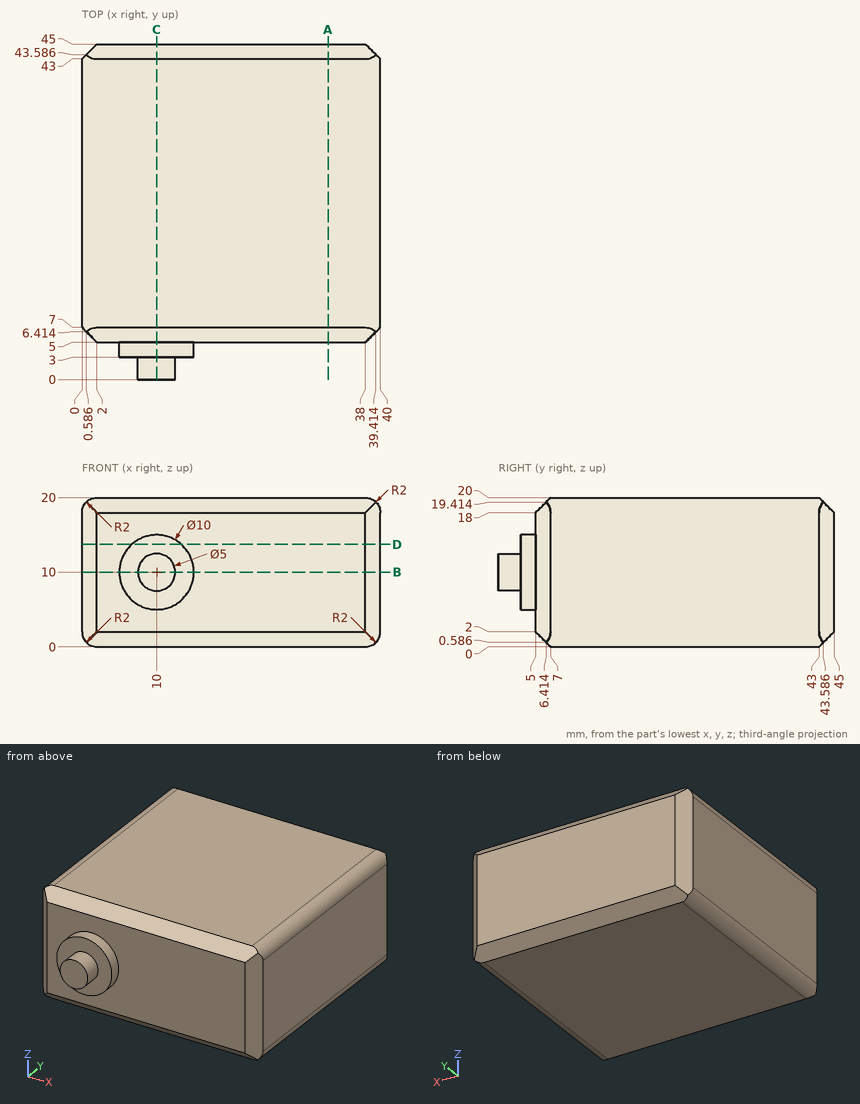
Input: dimensioned drawing with shaded views. Units: mm. Origin: part minimum x, y, z. Give positions to 0.01 mm unless a question says otherwise; leave off trailing zeros. Order: outer loops, then holes, each group sorted by start corner. A loop starts at its lowest first (then second) coordinate and runs counter-clockwise, first axis right, second up.
(1) Material intervals for line 1 along Y through (x, z) = (29.5, 17.75); line 2 along Y through (x, z) = (6.5, 10.5); line 3 along Z through (x, y) = (26, 43.5), sorted ascending.
(2) Section query B-B (z = 10). Return the cut outline in (x, y), plus the area to 3 significant figures.
(3) Section query D-D (z = 13.75). Return the cut outline in (x, y).
(4) Section query A-A (x = 33). Return the cut outline in (y, z).
(5) Section query C-C (x = 10). Return the cut outline in (y, z), plus the area to 3 significant figures.
(6) Contact query for flat-ended pins moving along their axis: P1, Ø10, axis at y = 25.5, z = 7, coming from the -X side; P2, Ø5, axis at x = 15.5, z = 12.5, coming from the -Y side. Output: stop coordinate, or through.
Outcome:
1. line 1: y = 5 to 45
1. line 2: y = 3 to 45
1. line 3: z = 0.5 to 19.5
2. outline: (0, 7) - (2, 5) - (5, 5) - (5, 3) - (7.5, 3) - (7.5, 0) - (12.5, 0) - (12.5, 3) - (15, 3) - (15, 5) - (38, 5) - (40, 7) - (40, 43) - (38, 45) - (2, 45) - (0, 43) - close
2. area: 1,630 mm2
3. outline: (0, 7) - (2, 5) - (6.69, 5) - (6.69, 3) - (13.31, 3) - (13.31, 5) - (38, 5) - (40, 7) - (40, 43) - (38, 45) - (2, 45) - (0, 43) - close
4. outline: (5, 2) - (7, 0) - (43, 0) - (45, 2) - (45, 18) - (43, 20) - (7, 20) - (5, 18) - close
5. outline: (0, 7.5) - (3, 7.5) - (3, 5) - (5, 5) - (5, 2) - (7, 0) - (43, 0) - (45, 2) - (45, 18) - (43, 20) - (7, 20) - (5, 18) - (5, 15) - (3, 15) - (3, 12.5) - (0, 12.5) - close
5. area: 827 mm2
6. P1: stops at x = 0
6. P2: stops at y = 3
